Design review of the part shown in the three views and the two pictorial views. Dimensions are in mm from the part's minimum x, y and z. A direction names the side the tool comes from. Coordinates: 2 decimals unless noted, no trailing zeros. Loops run counter-clockwise (first coordinate to the right, second up) from the corner with the lowest first, then second, coordinate; pieces in that order, holes last. Notation, with made-up numbers: (11, 0.5) -> (32, 0.5) arc R10 cw to (32, 8.5) -> close; hole circle Ø5 at (51.25, 68). An arc over 180 degrees is marked (long way). Answer in a Markdown table with one row per item.
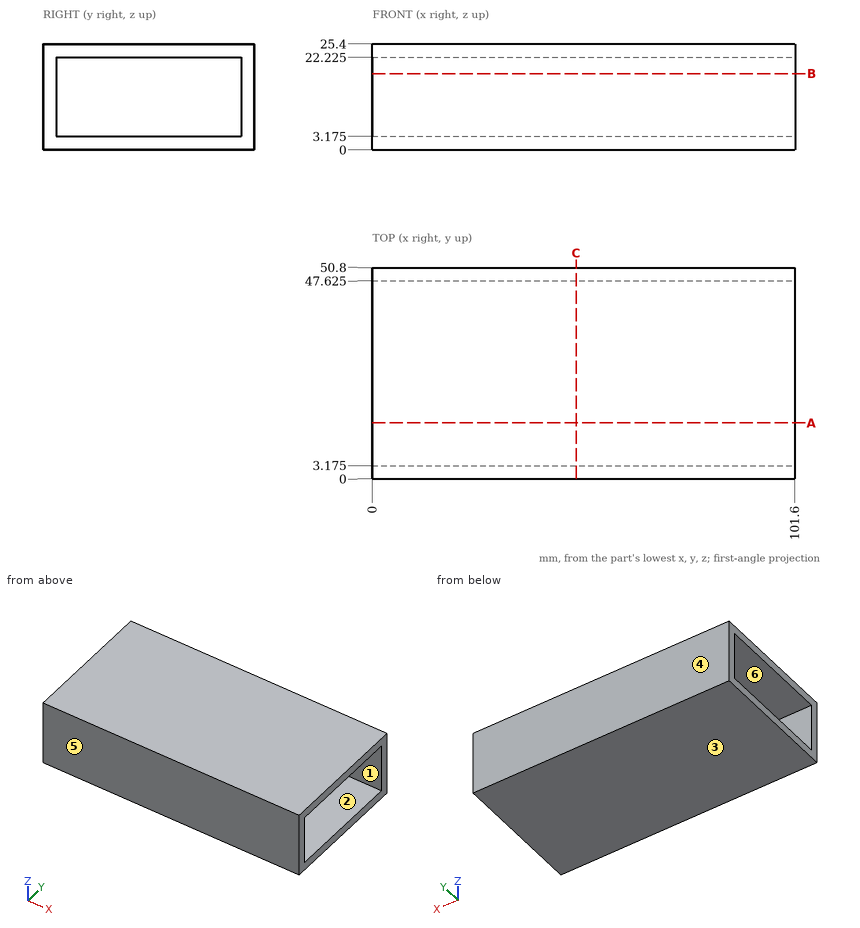
Item 1: Insertion check: pin 1 (9.5 mm diameter, centred on x = 46, z = 12.5, fed in from -Y); pin 2 (12 mm diameter, centred on y = 10.5, z = 10.5, fed in from -X). Each pin has a flat end and moves straight along its axis. Give the tip position at first contact, or say it passes through.
Worked answers:
| item | result |
|---|---|
| pin 1 | y = 0 |
| pin 2 | through |
Item 2: For L1, parallel to Z at x = 30, y = 11.5 (3 decimals); L2, parallel to Y at x = 74.5, z = 7 (3 decimals), list the stretches that pass through material, from the lowest coordinate up.
Worked answers:
| item | result |
|---|---|
| L1 | 0 to 3.175, 22.225 to 25.4 |
| L2 | 0 to 3.175, 47.625 to 50.8 |
Item 3: For the marked faces 5 and 6, list the 3-axis set-ups (+Z, -Z, +X, -X, +Y, -Y) from which the entire face can be reached by the end or side of a thin tool; tool diameter is ignored.
Worked answers:
| item | result |
|---|---|
| face 5 | +Z, -Z, +X, -X, -Y |
| face 6 | +X, -X |
Item 4: The part is to be moulded in two halves that separate along Y. For the marked faces 1, 2, 3 and 4, say which applies: +Y half, -Y half, draft (parallel to the pull), parting line (faces both ways), or undercut.
Worked answers:
| item | result |
|---|---|
| face 1 | undercut |
| face 2 | undercut |
| face 3 | draft |
| face 4 | +Y half |
Item 5: Take a section at C-C, the plane x = 49. State the section outline as (y, z) points (3 decimals), and give its area (3 significant figures).
Worked answers:
| item | result |
|---|---|
| outline | (0, 0) -> (50.8, 0) -> (50.8, 25.4) -> (0, 25.4) -> close; hole (3.175, 3.175) -> (47.625, 3.175) -> (47.625, 22.225) -> (3.175, 22.225) -> close |
| area | 444 mm² |
Item 6: Take a section at A-A, the plane y = 13.5. State the section outline as (x, z) points (3 decimals).
Worked answers:
| item | result |
|---|---|
| outline | (0, 0) -> (101.6, 0) -> (101.6, 3.175) -> (0, 3.175) -> close; (0, 22.225) -> (101.6, 22.225) -> (101.6, 25.4) -> (0, 25.4) -> close |
Item 7: Take a section at B-B, the plane z = 18.25. State the section outline as (x, y) points (3 decimals), and give its area (3 significant figures).
Worked answers:
| item | result |
|---|---|
| outline | (0, 0) -> (101.6, 0) -> (101.6, 3.175) -> (0, 3.175) -> close; (0, 47.625) -> (101.6, 47.625) -> (101.6, 50.8) -> (0, 50.8) -> close |
| area | 645 mm² |
